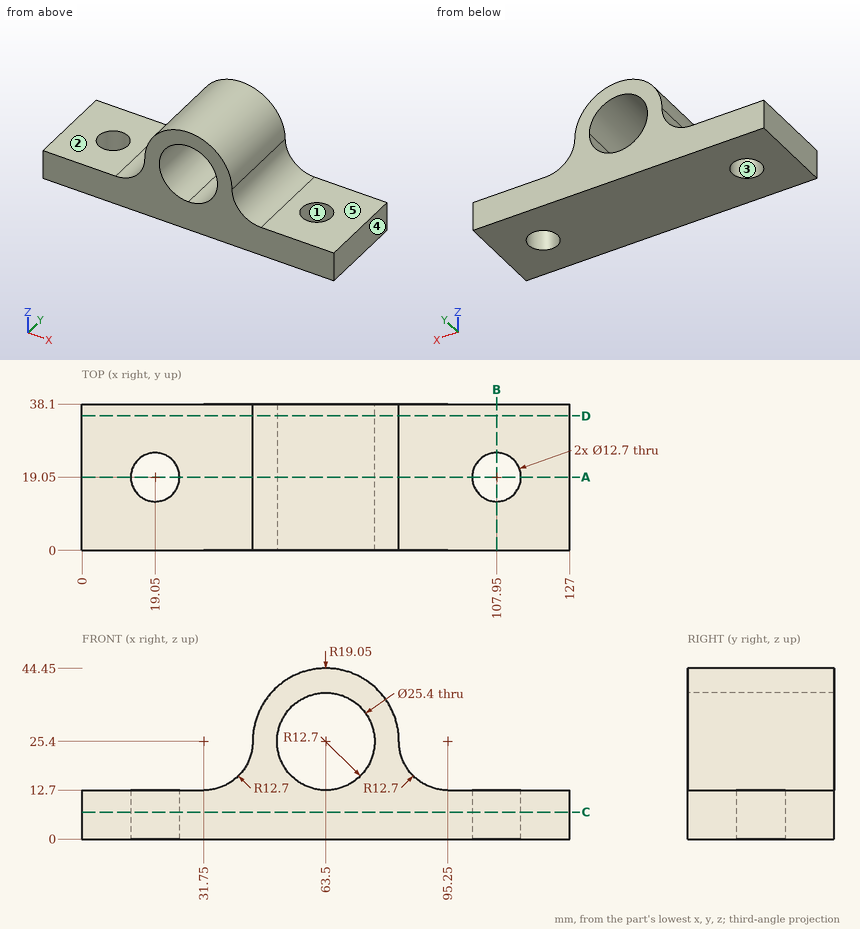
Here's the drawing with two shaded views (mm, measured from the low corner). I have some questions. A direction names the side the tool comes from. Coordinates: 2 decimals unless noted, no trailing zeros. Order: outer loops, then holes, each group sorted by start corner. A loop starts at its lowest first (then second) coordinate and runs counter-clockwise, first axis right, second up.
Item 1: Thinking about a two-plate mould opening in X: for the marked faces 3, 4 and 5, which applies, pulls with the +X half, pulls with the -X half, needs draft (parallel to the pull), parting line crosses it, or undercut?
Response values:
face 3: undercut
face 4: pulls with the +X half
face 5: needs draft
Item 2: Which directions (+Z, -Z, +X, -X, +Y, -Y) give clear straight access to the entire face, cutting with the end or side of a thin tool? Please do the marked faces 1 and 2.
Response values:
face 1: +Z, -Z
face 2: +Z, -X, +Y, -Y
Item 3: If we section it at D-D, the plane y = 35: List the corners of the cut face in (x, z) for me.
Response values:
outline: (0, 0) - (127, 0) - (127, 12.7) - (95.25, 12.7) arc R12.7 cw to (82.55, 25.4) arc R19.05 ccw to (44.45, 25.4) arc R12.7 cw to (31.75, 12.7) - (0, 12.7) - close; hole circle Ø25.4 at (63.5, 25.4)
Item 4: If we section it at B-B, the plane x = 107.95: List the corners of the cut face in (y, z) for me.
Response values:
outline: (0, 0) - (12.7, 0) - (12.7, 12.7) - (0, 12.7) - close; (25.4, 0) - (38.1, 0) - (38.1, 12.7) - (25.4, 12.7) - close
Item 5: I need wall thicknesses on probe 1 along X at (y, z) = (19, 5); probe 2 along Z at (x, y) = (63, 35); probe 3 along X at (y, z) = (18.5, 25.4). Which ranges of each line are inside material? Lowest first, please.
Response values:
probe 1: x = 0 to 12.7, 25.4 to 101.6, 114.3 to 127
probe 2: z = 0 to 12.71, 38.09 to 44.44
probe 3: x = 44.45 to 50.8, 76.2 to 82.55
Item 6: If we section it at A-A, the plane y = 19.05: List the corners of the cut face in (x, z) for me.
Response values:
outline: (0, 0) - (12.7, 0) - (12.7, 12.7) - (0, 12.7) - close; (25.4, 0) - (101.6, 0) - (101.6, 12.7) - (95.25, 12.7) arc R12.7 cw to (82.55, 25.4) arc R19.05 ccw to (44.45, 25.4) arc R12.7 cw to (31.75, 12.7) - (25.4, 12.7) - close; (114.3, 0) - (127, 0) - (127, 12.7) - (114.3, 12.7) - close; hole circle Ø25.4 at (63.5, 25.4)
Item 7: If we section it at C-C, the plane z = 7: List the corners of the cut face in (x, y) for me.
Response values:
outline: (0, 0) - (127, 0) - (127, 38.1) - (0, 38.1) - close; hole circle Ø12.7 at (19.05, 19.05); hole circle Ø12.7 at (107.95, 19.05)
Item 8: I'm going to push flat-ended pins straight in: pin 1 Ø2 at (y, z) = (17.5, 19.5) entering from +X; pin 2 Ø2 at (y, z) = (13.5, 29.5) entering from +X; pin 3 Ø12 at (y, z) = (29.5, 39.5) entering from -X. Where does each tip first touch, or does it pass through?
Response values:
pin 1: stops at x = 84.59
pin 2: stops at x = 82.3
pin 3: stops at x = 46.26
